Work out the finished part from the listing and answer in its coordinate system (mm). Round coordinates to 2 decimals unless told otherwise and drop trailing zeros. Return JSON: item names as keys, results as strings.
from build123d import *

# Parameters (mm, degrees)
F0_W     = 90.78
F0_H     = 17.7202104645
F1_DEPTH = 3
F3_D     = 6.6
F5_DEPTH = 25


with BuildPart() as f1:
    # F0 (on Top) → F1 (new body)
    with BuildSketch(Plane.XY):
        Polygon((-52.19, 13.3601052323), (-52.19, 8.8601052323), (38.59, 8.8601052323), (38.59, 13.3601052323), (38.59, 17.8601052323), (-52.19, 17.8601052323), align=None)
        with Locations((-6.8, 0)):
            Rectangle(F0_W, F0_H)
        Polygon((-42.115, 5.8601052323), (-37.04, 2.9300526161), (-37.04, -2.9300526161), (-42.115, -5.8601052323), (-47.19, -2.9300526161), (-47.19, 2.9300526161), align=None, mode=Mode.SUBTRACT)
        Polygon((-30.005, 4.6592166724), (-25.97, 2.3296083362), (-25.97, -2.3296083362), (-30.005, -4.6592166724), (-34.04, -2.3296083362), (-34.04, 2.3296083362), align=None, mode=Mode.SUBTRACT)
        Polygon((-19.845, 3.6084391824), (-16.72, 1.8042195912), (-16.72, -1.8042195912), (-19.845, -3.6084391824), (-22.97, -1.8042195912), (-22.97, 1.8042195912), align=None, mode=Mode.SUBTRACT)
        Polygon((-10.92, 3.2331615075), (-8.12, 1.6165807537), (-8.12, -1.6165807537), (-10.92, -3.2331615075), (-13.72, -1.6165807537), (-13.72, 1.6165807537), align=None, mode=Mode.SUBTRACT)
        Polygon((-2.56, 2.9560333783), (0, 1.4780166891), (0, -1.4780166891), (-2.56, -2.9560333783), (-5.12, -1.4780166891), (-5.12, 1.4780166891), align=None, mode=Mode.SUBTRACT)
        Polygon((5.06, 2.3786831091), (7.12, 1.1893415545), (7.12, -1.1893415545), (5.06, -2.3786831091), (3, -1.1893415545), (3, 1.1893415545), align=None, mode=Mode.SUBTRACT)
        Polygon((11.68, 1.8013328399), (13.24, 0.9006664199), (13.24, -0.9006664199), (11.68, -1.8013328399), (10.12, -0.9006664199), (10.12, 0.9006664199), align=None, mode=Mode.SUBTRACT)
        Polygon((17.595, 1.5646192295), (18.95, 0.7823096148), (18.95, -0.7823096148), (17.595, -1.5646192295), (16.24, -0.7823096148), (16.24, 0.7823096148), align=None, mode=Mode.SUBTRACT)
        Polygon((23.1, 1.3279056191), (24.25, 0.6639528096), (24.25, -0.6639528096), (23.1, -1.3279056191), (21.95, -0.6639528096), (21.95, 0.6639528096), align=None, mode=Mode.SUBTRACT)
        Polygon((28.15, 1.0392304845), (29.05, 0.5196152423), (29.05, -0.5196152423), (28.15, -1.0392304845), (27.25, -0.5196152423), (27.25, 0.5196152423), align=None, mode=Mode.SUBTRACT)
        Polygon((32.82, 0.8891194146), (33.59, 0.4445597073), (33.59, -0.4445597073), (32.82, -0.8891194146), (32.05, -0.4445597073), (32.05, 0.4445597073), align=None, mode=Mode.SUBTRACT)
    extrude(amount=F1_DEPTH)

    # F3 (through all)
    with Locations(Plane.XY.offset(3)):
        with Locations((-47.19, 13.4951905284), (-29.19, 13.4951905284), (-15.8, 13.4951905284), (2.2, 13.4951905284), (15.59, 13.4951905284), (33.59, 13.4951905284)):
            Hole(F3_D / 2)

    # F4 (on face) → F5 (cut)
    with BuildSketch(Plane.XY.offset(3)):
        with BuildLine():
            Line((-29.1901885501, 16.795190523), (-47.1078067859, 16.794166775))
            ThreePointArc((-47.1078067859, 16.794166775), (-44.8276666613, 15.79939998), (-43.89, 13.4951905284))
            ThreePointArc((-43.89, 13.4951905284), (-44.8276666613, 11.1909810768), (-47.1078067859, 10.1962142818))
            Line((-47.1078067859, 10.1962142818), (-29.1901885501, 10.1951905338))
            ThreePointArc((-29.1901885501, 10.1951905338), (-32.49, 13.4951905284), (-29.1901885501, 16.795190523))
        make_face()
        with BuildLine():
            Line((2.1994360639, 16.7951904802), (-15.7178067781, 16.7941667748))
            ThreePointArc((-15.7178067781, 16.7941667748), (-13.4376666586, 15.7993999772), (-12.5, 13.4951905284))
            ThreePointArc((-12.5, 13.4951905284), (-13.4377971224, 11.1908473324), (-15.7181803424, 10.1962049959))
            Line((-15.7181803424, 10.1962049959), (2.1998131641, 10.1951905337))
            ThreePointArc((2.1998131641, 10.1951905337), (-1.0999999946, 13.4950019783), (2.1994360639, 16.7951904802))
        make_face()
        with BuildLine():
            Line((33.5074298033, 16.794157361), (15.6725701967, 16.794157361))
            ThreePointArc((15.6725701967, 16.794157361), (17.9524649891, 15.799265001), (18.89, 13.4951905284))
            ThreePointArc((18.89, 13.4951905284), (17.9524649891, 11.1911160558), (15.6725701967, 10.1962236958))
            Line((15.6725701967, 10.1962236958), (33.4736921866, 10.1972407876))
            ThreePointArc((33.4736921866, 10.1972407876), (30.2900431541, 13.5120670006), (33.5074298033, 16.794157361))
        make_face()
    extrude(amount=-F5_DEPTH, mode=Mode.SUBTRACT)


solid = f1.part
Item 1: Consider line 1 along X through (y, z) = (13.5, 2.4); line 2 along X through (y, z) = (11, 0.6); line 3 along Y through (x, z) = (4.5, 0.65). Determine where each line is inside the solid, lowest interval first. Write a range as [from, to].
Output:
{"line 1": "x = [-52.19, -50.49], [-25.89, -19.1], [5.5, 12.29], [36.89, 38.59]", "line 2": "x = [-52.19, -49.35], [-27.03, -17.96], [4.36, 13.43], [35.75, 38.59]", "line 3": "y = [-8.86, -2.06], [2.06, 11.13], [15.86, 17.86]"}
Item 2: Find section A-A (z = 1.5). State how many separate pieces and enclosed holes the cut face has, plus the area to 3 significant figures.
Output:
{"separate pieces": "1", "enclosed holes": "14", "area": "1,700 mm^2"}
Item 3: The mould has two halves that part along X. Classify faces 1 (the cylindrical face through (5.5, 13.6, 1.5)), 2 (the flat face through (-22.97, 0, 1)), 3 (the flat face through (-6, 17.86, 1)): pulls with the +X half, pulls with the -X half, needs draft (parallel to the pull), parting line crosses it, or undercut.
Output:
{"face 1": "undercut", "face 2": "undercut", "face 3": "needs draft"}
